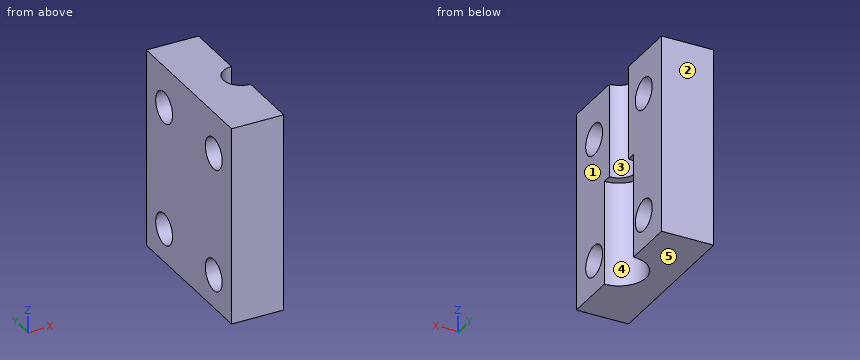
from build123d import *

# Parameters (mm, degrees)
EXTRUDE1_DEPTH = 10
EXTRUDE2_DEPTH = 9
SKETCH4_R      = 1.5
EXTRUDE3_DEPTH = 6


with BuildPart() as part:
    # Sketch1 → Extrude1 (new body)
    with BuildSketch(Plane.XY):
        with BuildLine():
            Line((0, 2.6), (0, 7.6))
            Line((0, 7.6), (-5, 7.6))
            Line((-5, 7.6), (-5, -7.6))
            Line((-5, -7.6), (0, -7.6))
            Line((0, -7.6), (0, -2.6))
            ThreePointArc((0, -2.6), (-2.6, 0), (0, 2.6))
        make_face()
    extrude(amount=EXTRUDE1_DEPTH)

    # Sketch2 → Extrude2 (add)
    with BuildSketch(Plane.XY.offset(10)):
        with BuildLine():
            Line((0, 1.7), (0, 7.6))
            Line((0, 7.6), (-5, 7.6))
            Line((-5, 7.6), (-5, -7.6))
            Line((-5, -7.6), (0, -7.6))
            Line((0, -7.6), (0, -1.7))
            ThreePointArc((0, -1.7), (-1.7, 0), (0, 1.7))
        make_face()
    extrude(amount=EXTRUDE2_DEPTH)

    # Sketch4 → Extrude3 (cut, through all)
    with BuildSketch(Plane.ZY.offset(5)):
        with Locations((3.175, 4.425)):
            Circle(SKETCH4_R)
        with Locations((15, 4.425)):
            Circle(SKETCH4_R)
        with Locations((15, -4.425)):
            Circle(SKETCH4_R)
        with Locations((3.175, -4.425)):
            Circle(SKETCH4_R)
    extrude(amount=-EXTRUDE3_DEPTH, mode=Mode.SUBTRACT)


solid = part.part
Geometry: final body of the model. Coordinates: model frame, mm. Face numbers are marked on the shaded views. A direction names the side the tool comes from. Round coordinates to 2 decimals unless told otherwise and drop trailing zeros. Order: outer loops, then holes, each group sorted by start corner. A loop starts at its lowest first (then second) coordinate and runs counter-clockwise, first axis right, second up.
Q1. Material intervals for probe 1 along Z at (x, y) = (-0.55, 4.5); probe 2 along Y at (x, z) = (-1.4, 15) (3 decimals); probe 3 along Y at (x, z) = (-1.2, 2.75), sorted ascending.
Result sheet:
probe 1: z = 0 to 1.68, 4.67 to 13.5, 16.5 to 19
probe 2: y = -7.6 to -5.925, -2.925 to -0.964, 0.964 to 2.925, 5.925 to 7.6
probe 3: y = -7.6 to -5.86, -2.99 to -2.31, 2.31 to 2.99, 5.86 to 7.6
Q2. Access query for the marked faces 4 and 5. Directions: +Z, -Z, +X, -X, +Y, -Y. A direction counts if a zero-diameter tool reaches every point of the face in a straight line with its end or side. Return the directions, or none.
Result sheet:
face 4: -Z, +X
face 5: -Z, +X, -X, +Y, -Y
Q3. Section A-A, the plane z = 15. Output: boundary loops of the cut face in (x, y) (3 decimals).
Result sheet:
outline: (-5, -7.6) - (0, -7.6) - (0, -5.925) - (-5, -5.925) - close; (-5, -2.925) - (0, -2.925) - (0, -1.7) arc R1.7 cw to (0, 1.7) - (0, 2.925) - (-5, 2.925) - close; (-5, 5.925) - (0, 5.925) - (0, 7.6) - (-5, 7.6) - close
Q4. Section C-C, the plane y = 5.25. Output: boundary loops of the cut face in (x, z), and give its area (3 significant figures).
Result sheet:
outline: (-5, 0) - (0, 0) - (0, 1.92) - (-5, 1.92) - close; (-5, 4.43) - (0, 4.43) - (0, 13.75) - (-5, 13.75) - close; (-5, 16.25) - (0, 16.25) - (0, 19) - (-5, 19) - close
area: 69.9 mm2
Q5. Section D-D, the plane x = -2.15. Output: boundary loops of the cut face in (y, z) (3 decimals).
Result sheet:
outline: (-7.6, 0) - (-1.462, 0) - (-1.462, 10) - (1.462, 10) - (1.462, 0) - (7.6, 0) - (7.6, 19) - (-7.6, 19) - close; hole circle Ø3 at (-4.425, 3.175); hole circle Ø3 at (-4.425, 15); hole circle Ø3 at (4.425, 3.175); hole circle Ø3 at (4.425, 15)
Q6. Section B-B, the plane x = -0.8. Output: boundary loops of the cut face in (y, z) (3 decimals), and give its area (3 significant figures).
Result sheet:
outline: (-7.6, 0) - (-2.474, 0) - (-2.474, 10) - (-1.5, 10) - (-1.5, 19) - (-7.6, 19) - close; (1.5, 10) - (2.474, 10) - (2.474, 0) - (7.6, 0) - (7.6, 19) - (1.5, 19) - close; hole circle Ø3 at (-4.425, 3.175); hole circle Ø3 at (-4.425, 15); hole circle Ø3 at (4.425, 3.175); hole circle Ø3 at (4.425, 15)
area: 184 mm2
Q7. Mould query, pull axis Y, two halves, no side actions, for the marked faces 1, 2 and 3. Classes: released by +Y, released by -Y, zero draft, split by the parting line, or undercut.
Result sheet:
face 1: zero draft
face 2: released by +Y
face 3: undercut
